```python
from build123d import *

# Parameters (mm, degrees)
SKETCH_1_R          = 2.25
EXTRUDE_1_DEPTH     = 2
FILLET_1_R          = 6
FILLET_2_R          = 3
CUT_EXTRUDE_1_DEPTH = 2
FILLET_3_R          = 2
CUT_EXTRUDE_2_DEPTH = 2
FILLET_4_R          = 2


with BuildPart() as part:
    # 草图1 → 凸台-拉伸1 (new body)
    # profile 1 of 2: a face of its own
    with BuildSketch(Plane.XY):
        with BuildLine():
            Line((50, 0), (0, 0))
            Line((0, 0), (0, -122.5))
            Line((0, -122.5), (2.75, -122.5))
            ThreePointArc((2.75, -122.5), (5, -120.25), (7.25, -122.5))
            Line((7.25, -122.5), (42.75, -122.5))
            ThreePointArc((42.75, -122.5), (45, -120.25), (47.25, -122.5))
            Line((47.25, -122.5), (50, -122.5))
            Line((50, -122.5), (50, 0))
        make_face()
        with Locations((5, -7.5)):
            Circle(SKETCH_1_R, mode=Mode.SUBTRACT)
        with Locations((45, -7.5)):
            Circle(SKETCH_1_R, mode=Mode.SUBTRACT)
    # profile 2 of 2: a face of its own
    with BuildSketch(Plane.XY):
        with BuildLine():
            Line((2.75, -122.5), (0, -122.5))
            Line((0, -122.5), (0, -130))
            Line((0, -130), (50, -130))
            Line((50, -130), (50, -122.5))
            Line((50, -122.5), (47.25, -122.5))
            ThreePointArc((47.25, -122.5), (45, -124.75), (42.75, -122.5))
            Line((42.75, -122.5), (7.25, -122.5))
            ThreePointArc((7.25, -122.5), (5, -124.75), (2.75, -122.5))
        make_face()
    extrude(amount=EXTRUDE_1_DEPTH)

    # 圆角1
    fillet_1_edges = [part.edges().sort_by_distance(p)[0] for p in [
        (0, 0, 1),
        (50, 0, 1),
        (50, -130, 1),
        (0, -130, 1),
    ]]
    fillet(fillet_1_edges, radius=FILLET_1_R)

    # 草图5 → 旋转1 (revolve)
    with BuildSketch(Plane(origin=(0, -33, 0), x_dir=(1, 0, 0), z_dir=(0, 1, 0))):
        Polygon((9, -2), (7, -2), (7.5, -11.5), (9, -11.5), align=None)
    revolve_1 = revolve(axis=Axis((9, -33, 2), (0, 0, 1)))

    # 镜向1: 旋转1 across plane
    add(revolve_1.mirror(Plane.ZY.offset(-25)))

    # 镜向1 at the second plane: 旋转1 across plane
    add(revolve_1.mirror(Plane.ZX.offset(-65)))

    # 镜向1 at the second plane copy 1 sket → 镜向1 at the second plane copy 1 (revolve)
    with BuildSketch(Plane(origin=(50, -97, 0), x_dir=(-1, 0, 0), z_dir=(0, -1, 0))):
        Polygon((9, -2), (7, -2), (7.5, -11.5), (9, -11.5), align=None)
    revolve(axis=Axis((41, -97, 2), (0, 0, 1)))

    # 圆角2
    fillet_2_edges = [part.edges().sort_by_distance(p)[0] for p in [
        (11, -33, 2),
        (11, -97, 2),
        (39, -33, 2),
        (39, -97, 2),
    ]]
    fillet(fillet_2_edges, radius=FILLET_2_R)

    # 草图7 → 切除-拉伸1 (cut)
    with BuildSketch(Plane.XY.offset(2)):
        Polygon((41, -15), (9, -15), (25, -33), align=None)
        Polygon((9, -65), (25, -83), (41, -65), (25, -47), align=None)
        Polygon((25, -97), (9, -115), (41, -115), align=None)
    extrude(amount=-CUT_EXTRUDE_1_DEPTH, mode=Mode.SUBTRACT)

    # 圆角3
    fillet_3_edges = [part.edges().sort_by_distance(p)[0] for p in [
        (25, -33, 1),
        (9, -15, 1),
        (41, -15, 1),
        (25, -83, 1),
        (9, -65, 1),
        (25, -47, 1),
        (41, -65, 1),
        (25, -97, 1),
        (41, -115, 1),
        (9, -115, 1),
    ]]
    fillet(fillet_3_edges, radius=FILLET_3_R)

    # 草图8 → 切除-拉伸2 (cut)
    with BuildSketch(Plane.XY.offset(2)):
        Polygon((5, -42.681670967), (5, -63.479202711), (23.486694883, -42.681670967), align=None)
        Polygon((45, -63.479202711), (26.513305117, -42.681670967), (45, -42.681670967), align=None)
        Polygon((45, -87.318329033), (45, -66.520797289), (26.513305117, -87.318329033), align=None)
        Polygon((5, -87.318329033), (5, -66.520797289), (23.486694883, -87.318329033), align=None)
    extrude(amount=-CUT_EXTRUDE_2_DEPTH, mode=Mode.SUBTRACT)

    # 圆角4
    fillet_4_edges = [part.edges().sort_by_distance(p)[0] for p in [
        (5, -87.318329033, 1),
        (5, -66.520797289, 1),
        (23.486694883, -87.318329033, 1),
        (45, -66.520797289, 1),
        (45, -87.318329033, 1),
        (26.513305117, -87.318329033, 1),
        (45, -63.479202711, 1),
        (26.513305117, -42.681670967, 1),
        (45, -42.681670967, 1),
        (5, -63.479202711, 1),
        (5, -42.681670967, 1),
        (23.486694883, -42.681670967, 1),
    ]]
    fillet(fillet_4_edges, radius=FILLET_4_R)


solid = part.part
```
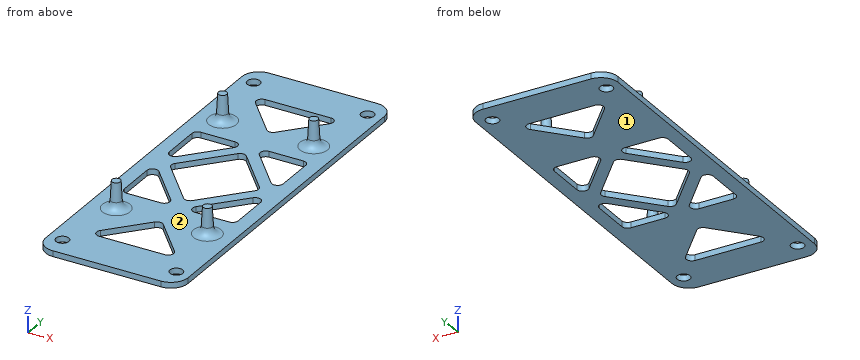
Model file for the job. Use its own axes, mm. Face numbers are marked on the shaded views. A direction names the side the tool comes from. Round coordinates to 2 decimals unless told otherwise and drop trailing zeros. Order: outer loops, then holes, each group sorted by start corner. A loop starts at its lowest first (then second) coordinate and runs counter-clockwise, first axis right, second up. Notation, with made-up numbers: M 77.5,31.25 L 102.5,31.25 A20 ccw 102.5,38.25 Z; hole C 27.25,48.5 d5. An arc over 180 degrees is marked long. Use CSV: the item, a comma, the result in double quotes.
Item 1: Pin check, flat tips, straight feed: pin 1 (5 mm diameter, centred on x = 5, y = -122.5, fed in from +Z); pin 2 (6 mm diameter, centred on x = 15, z = 7, fed in from -Y). Stop position of each tip, or through.
Worked answers:
pin 1,"z = 2"
pin 2,"through"
Item 2: Probe probe 1 along X at (y, z) = (-122.5, 0.5); probe 2 along Z at (x, y) = (32.5, -8); probe 3 along X at (y, z) = (-96.5, 5.5). List the from-to ranges inside material, lowest first.
Worked answers:
probe 1,"0 to 2.75, 7.25 to 42.75, 47.25 to 50"
probe 2,"0 to 2"
probe 3,"7.25 to 10.75, 39.25 to 42.75"
Item 3: Saw through at C-C (y = -53). List the corners of the cut face in (x, z).
Worked answers:
outline,"M 0,0 L 5,0 L 5,2 L 0,2 Z; M 14.31,0 L 19.67,0 L 19.67,2 L 14.31,2 Z; M 30.33,0 L 35.69,0 L 35.69,2 L 30.33,2 Z; M 45,0 L 50,0 L 50,2 L 45,2 Z"
Item 4: Saw through at A-A (x = 25). List the corners of the cut face in (y, z), plus the area to 3 significant figures.
Worked answers:
outline,"M -130,0 L -115,0 L -115,2 L -130,2 Z; M -98.01,0 L -81.99,0 L -81.99,2 L -98.01,2 Z; M -48.01,0 L -31.99,0 L -31.99,2 L -48.01,2 Z; M -15,0 L 0,0 L 0,2 L -15,2 Z"
area,"124 mm²"
Item 5: Which spindle directions (+Z, -Z, +X, -X, +Y, -Y) get a long thin tool onto all of the face, cutting with end or side? Do the marked faces 1 and 2. Say none if no direction does.
Worked answers:
face 1,"-Z, +X, -X, +Y, -Y"
face 2,"+Z"
Item 6: Saw through at B-B (y = -122.5). List the corners of the cut face in (x, z), plus the area to 3 significant figures.
Worked answers:
outline,"M 0,0 L 2.75,0 L 2.75,2 L 0,2 Z; M 7.25,0 L 42.75,0 L 42.75,2 L 7.25,2 Z; M 47.25,0 L 50,0 L 50,2 L 47.25,2 Z"
area,"82.0 mm²"
